from build123d import *

# Parameters (mm, degrees)
BASE_FLANGE1_DEPTH = 2.032
SKETCH6_R          = 2.921
CUT_EXTRUDE1_DEPTH = 2.54
HEM1_START         = -38.1
HEM1_DEPTH         = 76.2
HEM1_2_DEPTH       = 19.84375
HEM1_START_2       = 18.25625
HEM1_3_DEPTH       = 19.84375
CHAMFER2_SIZE      = 1.016


# Read off the part's stored shape, not the designer's step: Hem1
# Sheet-metal steps are written as plain solids
with BuildPart() as part:
    # Sketch1 → Base-Flange1 (new body)
    with BuildSketch(Plane(origin=(0, 0, 0), x_dir=(1, 0, 0), z_dir=(0, 1, 0))):
        Polygon((-15.08125, 38.1), (15.08125, 38.1), (15.08125, 18.25625), (-10.00125, 18.25625), (-10.00125, -18.25625), (15.08125, -18.25625), (15.08125, -38.1), (-15.08125, -38.1), align=None)
    extrude(amount=BASE_FLANGE1_DEPTH)

    # Sketch6 → Cut-Extrude1 (cut)
    with BuildSketch(Plane(origin=(0, 2.032, 0), x_dir=(1, 0, 0), z_dir=(0, 1, 0))):
        with Locations(Location((0, 29.36875, 0), (0, 0, 270))):
            Circle(SKETCH6_R)
        with Locations(Location((0, -29.36875, 0), (0, 0, 270))):
            Circle(SKETCH6_R)
    extrude(amount=-CUT_EXTRUDE1_DEPTH, mode=Mode.SUBTRACT)

    # Hem1 outline → Hem1 (cut)
    with BuildSketch(Plane.XY.offset(HEM1_START)):
        with BuildLine():
            Line((15.08125, 2.032), (14.536777241, 2.032))
            ThreePointArc((14.536777241, 2.032), (13.04925, 0.544472759), (11.01725, 0))
            Line((11.01725, 0), (15.08125, 0))
            Line((15.08125, 0), (15.08125, 2.032))
        make_face()
    extrude(amount=HEM1_DEPTH, mode=Mode.SUBTRACT)

    # Hem1 2 outline → Hem1 2 (add)
    with BuildSketch(Plane.XY.offset(HEM1_START)):
        with BuildLine():
            Line((7.364550996, 2.282459659), (9.190900498, 3.17322983))
            ThreePointArc((9.190900498, 3.17322983), (12.094045945, 5.787233731), (11.01725, 2.032))
            Line((11.01725, 2.032), (14.536777241, 2.032))
            ThreePointArc((14.536777241, 2.032), (11.159081554, 8.125524321), (7.364550996, 2.282459659))
        make_face()
    extrude(amount=HEM1_2_DEPTH)

    # Hem1 3 outline → Hem1 3 (add)
    with BuildSketch(Plane.XY.offset(HEM1_START_2)):
        with BuildLine():
            Line((7.364550996, 2.282459659), (9.190900498, 3.17322983))
            ThreePointArc((9.190900498, 3.17322983), (12.094045945, 5.787233731), (11.01725, 2.032))
            Line((11.01725, 2.032), (14.536777241, 2.032))
            ThreePointArc((14.536777241, 2.032), (11.159081554, 8.125524321), (7.364550996, 2.282459659))
        make_face()
    extrude(amount=HEM1_3_DEPTH)

    # Chamfer2
    chamfer2_edges = [part.edges().sort_by_distance(p)[0] for p in [
        (0, 2.032, -32.28975),
        (0, 2.032, 26.44775),
    ]]
    chamfer(chamfer2_edges, length=CHAMFER2_SIZE)


solid = part.part
Geometry check sheet. Reference: the model listing, model coordinates, mm. A direction names the side the tool comes from. Coordinates: 2 decimals unless noted, no trailing zeros. Order: outer loops, then holes, each group sorted by start corner. A loop starts at its lowest first (then second) coordinate and runs counter-clockwise, first axis right, second up. Notation, with made-up numbers: (-24, 65) -> (-20, 65) arc R20 ccw to (-20, 77) -> close; hole circle Ø5 at (-19.75, 23.5). An arc over 180 degrees is marked (long way). Use a Markdown table: item, result. Add a question column.
1. Cross-section at B-B (x = 0). Enter the section's corners in (y, z).
2. Material ranges on L1, parallel to Z at x = -4, y = 0.75; L2, parallel to Y at x = 6, z = 18.5; L3, parallel to X at y = 0.5, z = 1, recorded low to high.
3. Set-up check for faces 5 (the face through (-11, 0, -1)), 6 (the face through (-10.001, 1, 0)), 7 (the face through (8.26, 2.72, 28.04)): record each of +Z, -Z, +X, -X, +Y, -Y from which the full face is reachable in a straight line by a thin tool's end or side.
4. Cross-section at D-D (z = 0.5). Enter the section's corners in (x, y), and give its area (3 significant figures).
5. Go/stop test with a flat-tipped pin: pin 1 Ø3 at (y, z) = (2, 12.5) entering from +X. Record where the tip stops, or that it passes through.
6. Cross-section at A-A (x = 5). Enter the section's corners in (y, z), and give its area (3 significant figures).
7. Mould release check, pull along Z, two halves, no side actions. Record for faces 1 (the face through (3.3, 1.7, 38.1)), 2 (the face through (3.3, 1.7, -38.1)), 3 (the face through (8.26, 2.72, -28.32)), 4 (the face through (0.128, 0.515, -32.287)): pulls with the +Z half, pulls with the -Z half, needs draft (parallel to the pull), parting line crosses it, or undercut.
8. Cross-section at C-C (y = 7). Enter the section's corners in (x, z).
Filled sheet:
| question | item | result |
|---|---|---|
| 1 | outline | (0, -38.1) -> (2.03, -38.1) -> (2.03, -33.31) -> (1.02, -32.29) -> (0, -32.29) -> close; (0, -26.45) -> (1.02, -26.45) -> (2.03, -25.43) -> (2.03, -18.26) -> (0, -18.26) -> close; (0, 18.26) -> (2.03, 18.26) -> (2.03, 25.43) -> (1.02, 26.45) -> (0, 26.45) -> close; (0, 32.29) -> (1.02, 32.29) -> (2.03, 33.31) -> (2.03, 38.1) -> (0, 38.1) -> close |
| 2 | L1 | -38.1 to -18.26, 18.26 to 38.1 |
| 2 | L2 | 0 to 2.03 |
| 2 | L3 | -15.08 to -10 |
| 3 | face 5 | +Z, -Z, +X, -X, -Y |
| 3 | face 6 | +X, +Y, -Y |
| 3 | face 7 | +Z, -Z |
| 4 | outline | (-15.08, 0) -> (-10, 0) -> (-10, 2.03) -> (-15.08, 2.03) -> close |
| 4 | area | 10.3 mm2 |
| 5 | pin 1 | x = -10 |
| 6 | outline | (0, -38.1) -> (2.03, -38.1) -> (2.03, -18.26) -> (0, -18.26) -> close; (0, 18.26) -> (2.03, 18.26) -> (2.03, 38.1) -> (0, 38.1) -> close |
| 6 | area | 80.6 mm2 |
| 7 | face 1 | pulls with the +Z half |
| 7 | face 2 | pulls with the -Z half |
| 7 | face 3 | needs draft |
| 7 | face 4 | undercut |
| 8 | outline | (8.21, -38.1) -> (13.83, -38.1) -> (13.83, -18.26) -> (8.21, -18.26) -> close; (8.21, 18.26) -> (13.83, 18.26) -> (13.83, 38.1) -> (8.21, 38.1) -> close |
